Part model, mm, in its own coordinate system. A direction names the side the tool comes from. Coordinates: 2 decimals unless noted, no trailing zeros. Loops run counter-clockwise (first coordinate to the right, second up) from the corner with the lowest first, then second, coordinate; pieces in that order, holes last. Notation, with made-up numbers: (46, 55) - (98, 55) arc R35 cw to (98, 88) - close; hole circle Ø1 at (-31.5, 81). An arc over 180 degrees is marked (long way). Use a Markdown table: item, result. Add a question column.
1. 3-axis set-ups, long thin cutter, end or side, ignore diameter. For faces 4 (the flat face through (18, 1, -1.936)), 5 (the flat face through (-12, 1.65, -9)): which of +Z, -Z, +X, -X, +Y, -Y reach the whole face in a straight line?
2. Band-saw the part on B-B, the plane y = 0.5. Give the cut face in (x, z) (1 decimal), plus the area to 3 significant figures.
3. Band-saw the part on C-C, the plane x = 15. Give the cut face in (y, z).
4. Drop a flat-ended pin along its axis: pin 1 (0.8 mm diameter, centred on y = 0.5, z = 7, fed in from +X). Give the stop position or say it passes through.
5. Band-saw the part on A-A, the plane z = -18.51. Give the cut face in (x, y), plus the area to 3 significant figures.
6. Wall check: probe 1 along X at (y, z) = (0.55, -18.51); probe 2 along X at (y, z) = (1.3, -17.5); probe 3 along Z at (x, y) = (30.5, 0.45). Give the ranges that are in metal, low to high. Write a range as [from, to].
7. Pull direction Z, two halves, no side cores. Call faces 1 (the cylindrical face through (-19.21, 0.84, 7.37)), 2 (the flat face through (-20, 1, 10.764)), 3 (the flat face through (-12, 0, -9)): pulls with the +Z half, pulls with the -Z half, needs draft (parallel to the pull), parting line crosses it, or undercut.
Autodesk Inventor part; units mm, degrees
ref_plane "YZ Plane" through (0, 0, 0) normal (1, 0, 0) x (0, 1, 0)
ref_plane "XZ Plane" through (0, 0, 0) normal (0, 1, 0) x (-1, 0, 0)
ref_plane "XY Plane" through (0, 0, 0) normal (0, 0, 1) x (1, 0, 0)
sketch "Sketch1" plane through (0, 0, 0) normal (0, 1, 0) x (-1, 0, 0)
  line L0 (-33.6146, 10.7635) -> (42.5854, 10.7635)
  line L1 (42.5854, 10.7635) -> (42.5854, -22.2565)
  line L2 (42.5854, -22.2565) -> (-33.6146, -22.2565)
  line L3 (-33.6146, -22.2565) -> (-33.6146, 10.7635)
  line L4 (-33.6146, -22.2565) -> (-10.7151, -22.2565)
  line L5 (-33.6146, -8.8905) -> (-33.6146, -22.2565)
  line L6 (-33.6146, 10.7635) -> (-1.8646, 10.7635)
  line L7 (-1.8646, 10.7635) -> (-1.8646, -1.9365)
  line L8 (-1.8646, -1.9365) -> (-33.6146, -1.9365)
  line L9 (-33.6146, -1.9365) -> (-33.6146, 10.7635)
  point P0 (0, 0)
  dimension "d0" = 76.2
  dimension "d1" = 33.02
  dimension "d37" = 12.7
  dimension "d50" = 31.75
extrude "Extrusion1" add sketch "Sketch1" along normal blind 1.65 contours L0 L1 L2 L3 L8 L7
sketch "Sketch6" plane through (0, 1.65, 0) normal (0, 1, 0) x (1, 0, 0)
  line L0 (33.6146, 1.9365) -> (33.6146, 22.2565)
  line L1 (33.6146, 22.2565) -> (-42.5854, 22.2565)
  line L2 (-42.5854, 22.2565) -> (-42.5854, -10.7635)
  line L3 (-42.5854, -10.7635) -> (1.8646, -10.7635)
  circle A0 centre (-38.8262, 18.51) radius 1.5875
  circle A1 centre (29.8554, 18.51) radius 1.5875
  circle A2 centre (-20.6779, -6.763) radius 1.5875
  point P0 (0, 0)
  dimension "d39" = 3.175
  dimension "d40" = 3.175
  dimension "d41" = 3.175
  dimension "d42" = 21.9075
  dimension "d43" = 4.0005
  dimension "d44" = 3.7465
  dimension "d45" = 3.7465
  dimension "d46" = 3.7592
  dimension "d47" = 3.7592
extrude "Extrusion6" cut sketch "Sketch6" against normal blind 7.53
properties part number "InjectorBoard"
Geometry check:
| question | item | result |
|---|---|---|
| 1 | face 4 | +Z, +X, +Y, -Y |
| 1 | face 5 | +Z, -Z, +X, -X, +Y |
| 2 | outline | (-42.6, -22.3) - (33.6, -22.3) - (33.6, -1.9) - (1.9, -1.9) - (1.9, 10.8) - (-42.6, 10.8) - close; hole circle Ø3.2 at (-38.8, -18.5); hole circle Ø3.2 at (-20.7, 6.8); hole circle Ø3.2 at (29.9, -18.5) |
| 2 | area | 2,090 mm^2 |
| 3 | outline | (0, -22.26) - (1.65, -22.26) - (1.65, -1.94) - (0, -1.94) - close |
| 4 | pin 1 | stops at x = 1.86 |
| 5 | outline | (-42.59, 0) - (-40.41, 0) - (-40.41, 1.65) - (-42.59, 1.65) - close; (-37.24, 0) - (28.27, 0) - (28.27, 1.65) - (-37.24, 1.65) - close; (31.44, 0) - (33.61, 0) - (33.61, 1.65) - (31.44, 1.65) - close |
| 5 | area | 115 mm^2 |
| 6 | probe 1 | x = [-42.59, -40.41], [-37.24, 28.27], [31.44, 33.61] |
| 6 | probe 2 | x = [-42.59, -40.05], [-37.6, 28.63], [31.08, 33.61] |
| 6 | probe 3 | z = [-22.26, -19.96], [-17.06, -1.94] |
| 7 | face 1 | undercut |
| 7 | face 2 | pulls with the +Z half |
| 7 | face 3 | needs draft |
